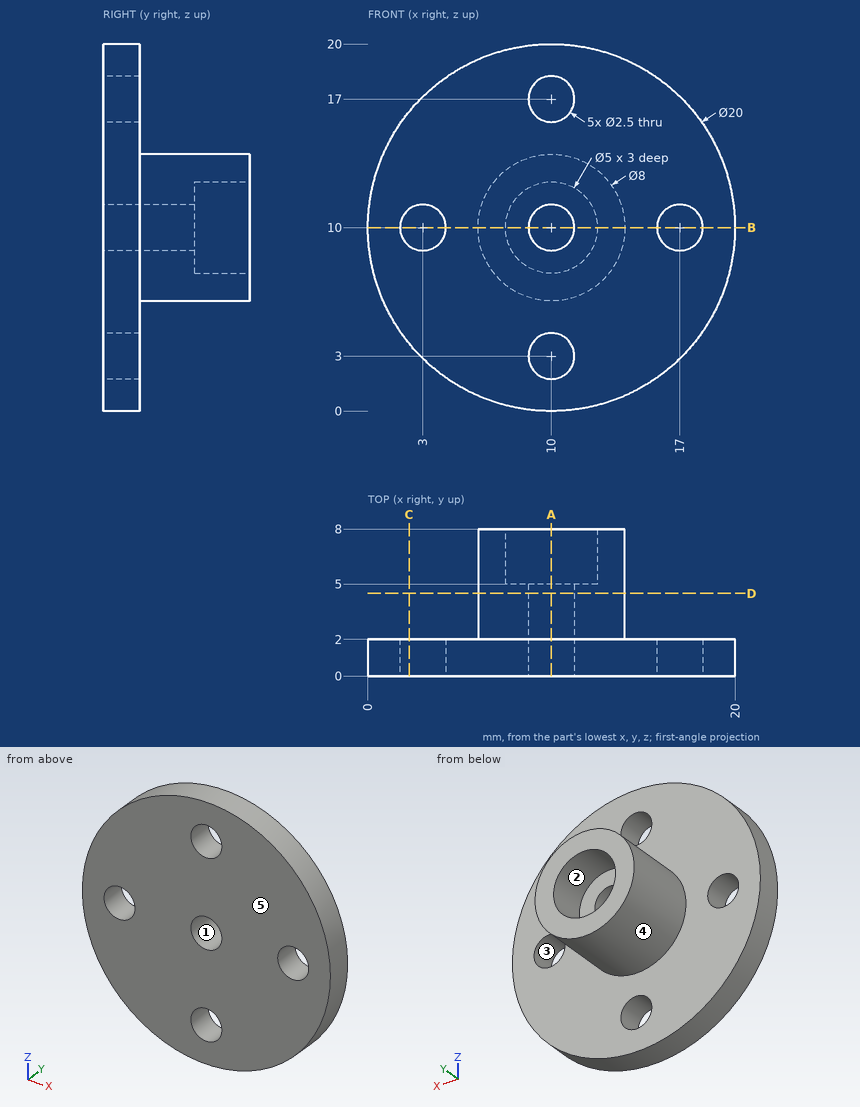
Geometry check sheet. Reference: drawing and pictorial views, mm from the part's lowest x, y, z. A direction names the side the tool comes from. Coordinates: 2 decimals unless noted, no trailing zeros. Order: outer loops, then holes, each group sorted by start corner. A loop starts at its lowest first (then second) coordinate and runs counter-clockwise, first axis right, second up.
1. Sectioned sample at A-A, the plane x = 10. Record the cut outline in (y, z), and give its area (3 significant figures).
Results found:
outline: (0, 0) - (2, 0) - (2, 1.75) - (0, 1.75) - close; (0, 4.25) - (2, 4.25) - (2, 6) - (8, 6) - (8, 7.5) - (5, 7.5) - (5, 8.75) - (0, 8.75) - close; (0, 11.25) - (5, 11.25) - (5, 12.5) - (8, 12.5) - (8, 14) - (2, 14) - (2, 15.75) - (0, 15.75) - close; (0, 18.25) - (2, 18.25) - (2, 20) - (0, 20) - close
area: 50.5 mm2
2. Scan lines: line 1 (X direction, y = 3, z = 10); line 2 (Z direction, x = 10, y = 7.1). Record each from-to range of solid material in increasing order.
Results found:
line 1: x = 6 to 8.75, 11.25 to 14
line 2: z = 6 to 7.5, 12.5 to 14
3. Sectioned sample at C-C, the plane x = 2.25. Record the cut outline in (y, z).
Results found:
outline: (0, 3.68) - (2, 3.68) - (2, 9) - (0, 9) - close; (0, 11) - (2, 11) - (2, 16.32) - (0, 16.32) - close
4. Release check for a two-part mould opening along Z. For the marked faces 3, 4 and 5 record: +Z half, -Z half, draft (parallel to the pull), parting line (faces both ways), or undercut.
Results found:
face 3: undercut
face 4: parting line
face 5: draft
5. Sectioned sample at D-D, the plane y = 4.5. Record the cut outline in (x, z).
Results found:
outline: circle Ø8 at (10, 10); hole circle Ø2.5 at (10, 10)
6. Go/stop test with flat-tipped pins: pin 1 Ø3 at (x, z) = (3, 10) entering from +Y; pin 2 Ø1 at (x, y) = (17.5, 1) entering from +Z; pin 3 Ø3 at (x, z) = (10, 10) entering from +Y. Record where each tip stops, or that it passes through.
Results found:
pin 1: stops at y = 2
pin 2: stops at z = 17.14
pin 3: stops at y = 5
7. Sectioned sample at B-B, the plane z = 10. Record the cut outline in (x, y), and give its area (3 significant figures).
Results found:
outline: (0, 0) - (1.75, 0) - (1.75, 2) - (0, 2) - close; (4.25, 0) - (8.75, 0) - (8.75, 5) - (7.5, 5) - (7.5, 8) - (6, 8) - (6, 2) - (4.25, 2) - close; (11.25, 0) - (15.75, 0) - (15.75, 2) - (14, 2) - (14, 8) - (12.5, 8) - (12.5, 5) - (11.25, 5) - close; (18.25, 0) - (20, 0) - (20, 2) - (18.25, 2) - close
area: 50.5 mm2
8. Set-up check for the marked faces 1 and 2: record each of +Z, -Z, +X, -X, +Y, -Y from which the full face is reachable in a straight line by a thin tool's end or side.
Results found:
face 1: +Y, -Y
face 2: +Y
